The listing builds one solid part. Answer for the finished solid, in the listing's coordinates (mm). Face numbers are marked on the shaded views. A direction names the side the tool comes from. Coordinates: 2 decimals unless noted, no trailing zeros. Loops run counter-clockwise (first coordinate to the right, second up) from the corner with the lowest first, then second, coordinate; pieces in that order, holes last. Notation, with made-up numbers: (30.25, 82) -> (52.25, 82) arc R23 cw to (52.25, 91) -> close; hole circle Ø3 at (28, 16.5). An arc over 180 degrees is marked (long way). Answer in a Markdown table with one row per item.
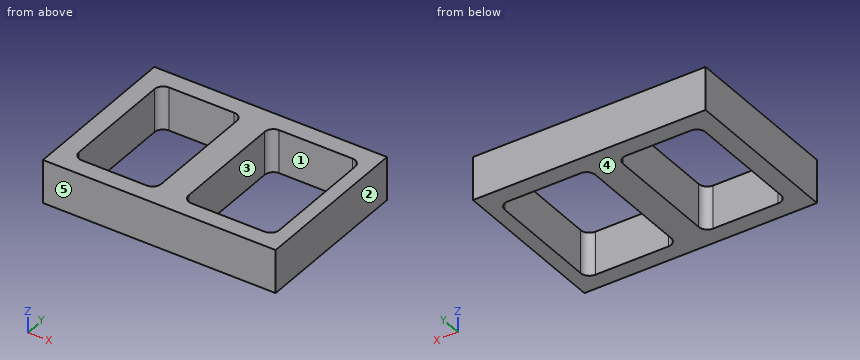
```python
from build123d import *

# Parameters (mm, degrees)
F0_W     = 134.455651
F0_H     = 94.536297
F1_DEPTH = 25
F2_W     = 47.540324
F2_H     = 74.032262
F3_DEPTH = 25
F2_W_2   = 52.258067
F2_H_2   = 74.395165
F4_DEPTH = 25
F5_R     = 5


with BuildPart() as f1:
    # F0 (on Top) → F1 (new body)
    with BuildSketch(Plane.XY):
        with Locations((0.090725, 0.090726)):
            Rectangle(F0_W, F0_H)
    extrude(amount=F1_DEPTH)

    # F2 (on face) → F3 (cut)
    with BuildSketch(Plane.XY.offset(25)):
        with Locations((-32.842743, 0)):
            Rectangle(F2_W, F2_H)
    extrude(amount=-F3_DEPTH, mode=Mode.SUBTRACT)

    # F2 (on face) → F4 (cut)
    with BuildSketch(Plane.XY.offset(25)):
        with Locations((-32.842743, 0)):
            Rectangle(F2_W, F2_H)
        with Locations((33.205647, -0.181451)):
            Rectangle(F2_W_2, F2_H_2)
    extrude(amount=-F4_DEPTH, mode=Mode.SUBTRACT)

    # F5
    f5_edges = [f1.edges().sort_by_distance(p)[0] for p in [
        (-56.612905, 37.016131, 12.5),
        (-9.072581, 37.016131, 12.5),
        (-56.612905, -37.016131, 12.5),
        (-9.072581, -37.016131, 12.5),
        (7.076613, -37.379034, 12.5),
        (7.076613, 37.016131, 12.5),
        (59.33468, 37.016131, 12.5),
        (59.33468, -37.379034, 12.5),
    ]]
    fillet(f5_edges, radius=F5_R)


solid = f1.part
```
Item 1: A cutting plane is placed at B-B, the plane x = -31.5. Determine the outline of the cut face in (y, z).
Findings below:
| item | result |
|---|---|
| outline | (-47.18, 0) -> (-37.02, 0) -> (-37.02, 25) -> (-47.18, 25) -> close; (37.02, 0) -> (47.36, 0) -> (47.36, 25) -> (37.02, 25) -> close |
Item 2: A cutting plane is placed at A-A, the plane y = 0. Determine the outline of the cut face in (x, z).
Findings below:
| item | result |
|---|---|
| outline | (-67.14, 0) -> (-56.61, 0) -> (-56.61, 25) -> (-67.14, 25) -> close; (-9.07, 0) -> (7.08, 0) -> (7.08, 25) -> (-9.07, 25) -> close; (59.33, 0) -> (67.32, 0) -> (67.32, 25) -> (59.33, 25) -> close |
Item 3: A cutting plane is placed at D-D, the plane x = 37. Determine the outline of the cut face in (y, z), plus the area to 3 significant figures.
Findings below:
| item | result |
|---|---|
| outline | (-47.18, 0) -> (-37.38, 0) -> (-37.38, 25) -> (-47.18, 25) -> close; (37.02, 0) -> (47.36, 0) -> (47.36, 25) -> (37.02, 25) -> close |
| area | 504 mm2 |
Item 4: A cutting plane is placed at C-C, the plane z = 14.5. Determine the outline of the cut face in (x, y), plus the area to 3 significant figures.
Findings below:
| item | result |
|---|---|
| outline | (-67.14, -47.18) -> (67.32, -47.18) -> (67.32, 47.36) -> (-67.14, 47.36) -> close; hole (-56.61, -32.02) arc R5 ccw to (-51.61, -37.02) -> (-14.07, -37.02) arc R5 ccw to (-9.07, -32.02) -> (-9.07, 32.02) arc R5 ccw to (-14.07, 37.02) -> (-51.61, 37.02) arc R5 ccw to (-56.61, 32.02) -> close; hole (7.08, -32.38) arc R5 ccw to (12.08, -37.38) -> (54.33, -37.38) arc R5 ccw to (59.33, -32.38) -> (59.33, 32.02) arc R5 ccw to (54.33, 37.02) -> (12.08, 37.02) arc R5 ccw to (7.08, 32.02) -> close |
| area | 5,350 mm2 |
Item 5: A tool of negligible diameter and unlimited length cuts with its end or side. For the marked faces 1 and 2, from which of +Z, -Z, +X, -X, +Y, -Y can it reach the whole face along a straight path? Write none if from no direction.
Findings below:
| item | result |
|---|---|
| face 1 | +Z, -Z |
| face 2 | +Z, -Z, +X, +Y, -Y |
Item 6: Determine the mould class of the marked faces 3, 4 and 5 for opening direction Y: +Y half, -Y half, draft (parallel to the pull), parting line (faces both ways), or undercut.
Findings below:
| item | result |
|---|---|
| face 3 | undercut |
| face 4 | draft |
| face 5 | -Y half |
Item 7: Find the intervals of material crossed by probe 1 along X at (y, z) = (32.5, 2.25); probe 2 along Y at (x, z) = (14.5, 6.75); probe 3 along X at (y, z) = (33, 22.5), in increasing order.
Findings below:
| item | result |
|---|---|
| probe 1 | x = -67.14 to -56.59, -9.1 to 7.1, 59.31 to 67.32 |
| probe 2 | y = -47.18 to -37.38, 37.02 to 47.36 |
| probe 3 | x = -67.14 to -56.52, -9.17 to 7.17, 59.24 to 67.32 |
